Job drawing, mm, ordinate dimensions from the low corner. One solid piece. Give positions to 0.01 mm unless a question says otherwise; leave off trailing zeros. Loops run counter-clockwise (first coordinate to the right, second up) from the corner with the lowest first, then second, coordinate; pieces in that order, holes last. Notation, with made-up numbers: M -27,52 L 28,52 A16 cw 28,80 Z; hole C -9.75,53.25 d6. An arc over 180 degrees is marked long. Put each result on its own line as item: value.
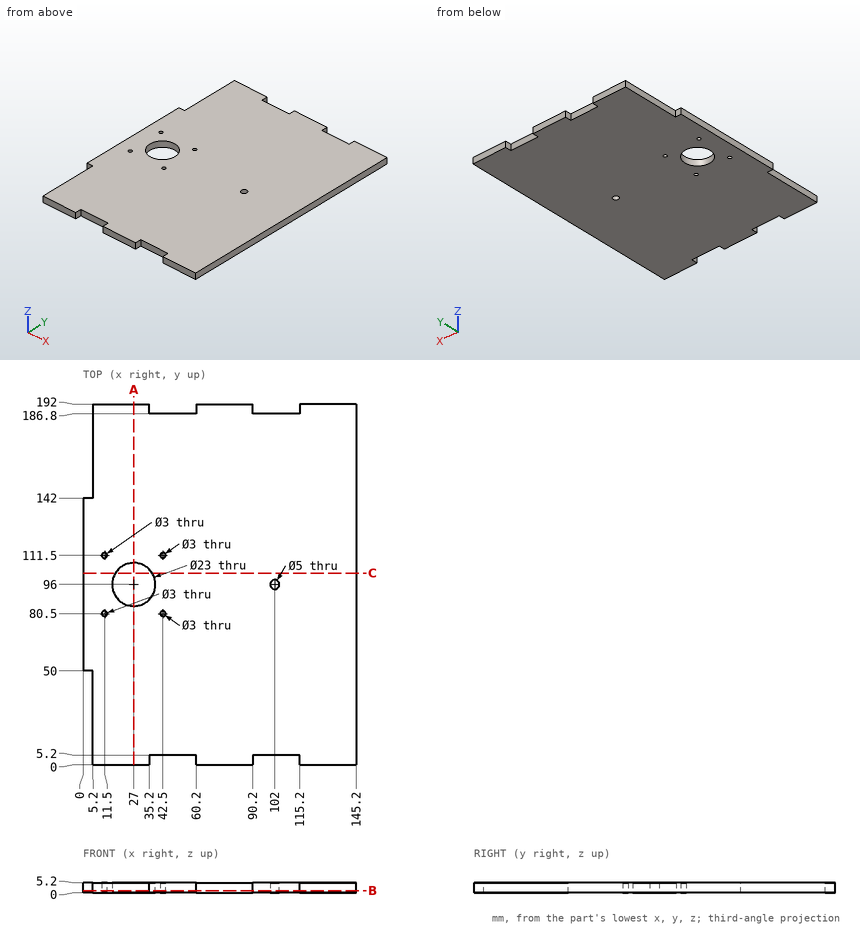
Q1. Drop flat-ended pins along their axis: pin 1 Ø3 at (y, z) = (19.5, 2.5) entering from -X; pin 2 Ø3 at (x, y) = (102, 96) entering from -Z; pin 3 Ø1.6 at (x, z) = (1.5, 3.5) entering from -Y. Give the stop position or say it passes through.
Here are the results:
pin 1: x = 5.2
pin 2: through
pin 3: y = 50
Q2. Probe line 1 (Y direction, x = 11.5, z = 1.7); line 2 (X direction, y = 111.5, z = 3.1); line 3 (Y direction, x = 27.5, z = 2.5). List the from-to ranges inside material, lowest first. Write a range as from..to.
Here are the results:
line 1: 0..79, 82..110, 113..192
line 2: 0..10, 13..41, 44..145.2
line 3: 0..84.51, 107.49..192
Q3. Slice it at C-C (y = 102). List the corners of the cut face in (x, z).
Here are the results:
outline: M 0,0 L 17.19,0 L 17.19,5.2 L 0,5.2 Z; M 36.81,0 L 145.2,0 L 145.2,5.2 L 36.81,5.2 Z
Q4. Slice it at B-B (z = 1.1). State how many separate pieces and enclosed holes the cut face has, and give its area (3 significant figures).
Here are the results:
separate pieces: 1
enclosed holes: 6
area: 26,400 mm²
Q5. Slice it at A-A (x = 27). List the corners of the cut face in (y, z).
Here are the results:
outline: M 0,0 L 84.5,0 L 84.5,5.2 L 0,5.2 Z; M 107.5,0 L 192,0 L 192,5.2 L 107.5,5.2 Z
